For this review, take the finished solid that the model builds, in its own axes (mm). A direction names the side the tool comes from. Give positions to 0.01 mm unless a question says otherwise; leave off trailing zeros. Write each loop counter-clockwise with the first axis right and the second up, starting at its lowest first coordinate (ties: lowest second). Pieces come first, ordered by that corner, then holes. Notation, with made-up numbers: M 11.25,35 L 44.25,35 A20 cw 44.25,54 Z; hole C 54.5,27 d6. An arc over 180 degrees is marked long. One line per item, written item: value. Start each with the question number.
Item 1: Clearance check with flat-ended pins moving along their axes: pin 1 Ø1 at (x, z) = (-10.5, 3) entering from -Y; pin 2 Ø1 at (x, z) = (0.5, 0) entering from -Y; pin 3 Ø1 at (y, z) = (44, -1) entering from -X; pin 4 Ø4 at (x, y) = (-19, 4) entering from +Z. State where each tip first meets the part, or that it passes through.
Item 2: To check wall thickness, follow probe 1 along Z at (x, y) = (-10, 38); probe 2 along X at (y, z) = (54.5, 1.6). State the ranges of each line that lie inside material, in increasing order.
Item 3: Consider section A-A, the plane z = -0.75. Write out the cut boundary in (x, y), and give its area (3 significant figures).
Item 4: Consider section C-C, the plane y = 55. Write out the cut boundary in (x, z), and give its area (3 significant figures).
Item 5: Consider section B-B, the plane x = -21.5. Write out the cut boundary in (y, z), and give its area (3 significant figures).
Item 6: Tool access review of faces 1 (the face through (1, 0, 1)), 2 (the face through (0, 39, -1)), 3 (the face through (2, 39, 1)), 4 (the face through (0, 39, 3)): name each direction out of +Z, -Z, +X, -X, +Y, -Y from which nothing blocks a thin tool from reaching the whole face with its end or side.
Item 7: Consider section D-D, the plane y = 74.5. Write out the cut boundary in (x, z), and give its area (3 significant figures).
```python
from build123d import *

# Parameters (mm, degrees)
F1_DEPTH  = 2
F1_FACE_W = 80
F1_FACE_H = 2
F2_DEPTH  = 2
F3_W      = 2
F3_H      = 80
F4_DEPTH  = 2
F5_DEPTH  = 4


with BuildPart() as f1:
    # F0 (on Top) → F1 (new body)
    with BuildSketch(Plane.XY):
        Polygon((-25, -5), (0, 0), (0, 80), align=None)
    extrude(amount=F1_DEPTH)

    # F1_face (on face) → F2 (join)
    with BuildSketch(Plane(origin=(0, 40, 1), x_dir=(0, 1, 0), z_dir=(1, 0, 0))):
        Rectangle(F1_FACE_W, F1_FACE_H)
    extrude(amount=F2_DEPTH)

    # F3 (on face) → F4 (join)
    with BuildSketch(Plane.XY.offset(2)):
        with Locations((1, 40)):
            Rectangle(F3_W, F3_H)
    extrude(amount=F4_DEPTH)

    # F3 (on face) → F5 (join)
    with BuildSketch(Plane.XY.offset(2)):
        with Locations((1, 40)):
            Rectangle(F3_W, F3_H)
    extrude(amount=-F5_DEPTH)


solid = f1.part
```
Model answer:
1. pin 1: passes through
1. pin 2: stops at y = 0
1. pin 3: stops at x = 0
1. pin 4: stops at z = 2
2. probe 1: z = 0 to 2
2. probe 2: x = -7.5 to 2
3. outline: M 0,0 L 2,0 L 2,80 L 0,80 Z
3. area: 160 mm2
4. outline: M -7.35,0 L 0,0 L 0,-2 L 2,-2 L 2,4 L 0,4 L 0,2 L -7.35,2 Z
4. area: 26.7 mm2
5. outline: M -4.3,0 L 6.9,0 L 6.9,2 L -4.3,2 Z
5. area: 22.4 mm2
6. face 1: +Z, -Z, +X, -Y
6. face 2: -Z, -X, +Y, -Y
6. face 3: +Z, -Z, +X, +Y, -Y
6. face 4: +Z, -X, +Y, -Y
7. outline: M -1.62,0 L 0,0 L 0,-2 L 2,-2 L 2,4 L 0,4 L 0,2 L -1.62,2 Z
7. area: 15.2 mm2
